For this review, take the finished solid that the model builds, in its own axes (mm). Face numbers are marked on the shaded views. A direction names the side the tool comes from. Coordinates: 2 decimals unless noted, no trailing zeros. Write each loop counter-clockwise with the first axis right and the second up, starting at its lowest first coordinate (ties: lowest second). Pieces come first, ordered by that corner, then holes. Notation, with made-up numbers: (69, 47.5) - (91, 47.5) arc R20 cw to (91, 70.5) - close; hole circle Ø3 at (81, 15). An arc over 180 degrees is marked (long way). Write each question's results on one line, items separated by ' | '.
Autodesk Inventor part; units mm, degrees
ref_plane "YZ Plane" through (0, 0, 0) normal (1, 0, 0) x (0, 1, 0)
ref_plane "XZ Plane" through (0, 0, 0) normal (0, 1, 0) x (-1, 0, 0)
ref_plane "XY Plane" through (0, 0, 0) normal (0, 0, 1) x (1, 0, 0)
sketch "Boceto1" plane through (0, 0, 0) normal (0, 0, 1) x (1, 0, 0)
  line L0 (64, 24) -> (64, 0)
  line L1 (0, 0) -> (0, 24)
  line L2 (0, 0) -> (0, 24) construction
  line L3 (40, 7) -> (40, 16)
  line L4 (64, 0) -> (64, 24)
  line L5 (0, 24) -> (0, 0)
  line L6 (64, 0) -> (64, 16)
  line L7 (40, 16) -> (24, 16)
  line L8 (0, 16) -> (0, 0)
  line L9 (24, 16) -> (40, 16)
  line L10 (64, 16) -> (64, 7)
  line L11 (0, 7) -> (0, 16)
  line L12 (48, 0) -> (48, 7)
  line L13 (16, 7) -> (16, 0)
  line L14 (24, 16) -> (24, 7)
  line L15 (48, 7) -> (40, 7)
  line L16 (24, 7) -> (16, 7)
  arc A0 (45.1449, 45.122) -> (18.8863, 45.1669) centre (32, 36) ccw
  circle A1 centre (32, 36) radius 8
  line L17 (64, 24) -> (59.8026, 24)
  line L18 (4.09, 24) -> (0, 24)
  line L19 (64, 0) -> (48, 0)
  line L20 (16, 0) -> (0, 0)
  line L21 (0, 0) -> (16, 0)
  line L22 (48, 0) -> (60.5696, 0)
  line L23 (0, 0) -> (16, 0)
  line L24 (48, 0) -> (64, 0)
  line L25 (0, 0) -> (16, 0)
  line L26 (48, 0) -> (64, 0)
  line L27 (4.09, 24) -> (18.8863, 45.1669)
  line L28 (45.1449, 45.122) -> (59.8026, 24)
  line L29 (16, 0) -> (48, 0)
  line L30 (0, 0) -> (64, 0)
  line L31 (64, 0) -> (64, 24)
  line L32 (32.0546, 51.9999) -> (31.9454, 51.9999)
  line L33 (0, 24) -> (0, 0)
  line L34 (0, 0) -> (64, 0)
  line L35 (64, 0) -> (64, 53.4326)
  line L36 (64, 53.4326) -> (0, 53.4326)
  line L37 (0, 53.4326) -> (0, 0)
  circle A2 centre (32, 36) radius 8
  point P0 (30.2848, 0)
  dimension "d6" = 24
  dimension "d9" = 32
  dimension "d10" = 16
  dimension "d11" = 9
sketch "Boceto2" plane through (0, 0, 0) normal (1, 0, 0) x (0, 1, 0)
  point P0 (0, 0)
sketch "Boceto3" plane through (0, 0, 0) normal (1, 0, 0) x (0, 1, 0)
  point P0 (0, 0)
sketch "Boceto4" plane through (0, 0, 0) normal (1, 0, 0) x (0, 1, 0)
  line L0 (0, 0) -> (0, -144)
  line L1 (0, -144) -> (36, -144)
  line L2 (0, -144) -> (16, -144)
  line L3 (16, -118) -> (16, -22)
  line L4 (16, 0) -> (0, 0)
  line L5 (0, 0) -> (0, -144)
  line L6 (36, -144) -> (16, -144)
  line L7 (16, -118) -> (52, -118)
  line L8 (52, -118) -> (52, -128)
  line L9 (36, -144) -> (52, -128)
  line L10 (52, 0) -> (16, 0)
  line L11 (16, -22) -> (52, -22)
  line L12 (52, -22) -> (52, 0)
  line L13 (52, -128) -> (52, -118)
  line L14 (52, -22) -> (52, 0)
  dimension "d15" = 144
  dimension "d17" = 16
  dimension "d22" = 22
extrude "Extrusión1" add sketch "Boceto4" along normal blind 64
extrude "Extrusión3" cut sketch "Boceto1" against normal blind 100 contours L17 L28 A0 L27 L18 L37 L36 L35
extrude "Extrusión4" cut sketch "Boceto1" against normal blind 100 contours A1
extrude "Extrusión5" cut sketch "Boceto1" against normal blind 144 contours L29 L13 L16 L14 L7 L3 L15 L12
fillet "Empalme1" radius 3 2 edges at (59.8026, 24, -11) (4.09, 24, -11)
properties part number "Pieza2 Base" material "Hierro, fundido"
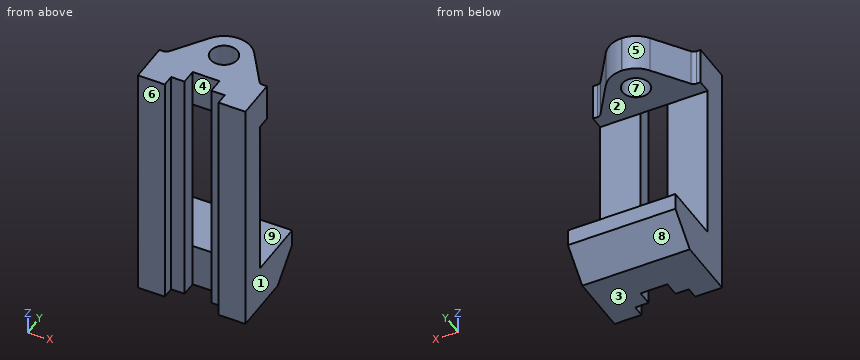
Q1. Take a section at C-C on y = 29.5. State the section outline as (x, z) points, plus the area to 3 significant figures.
Results found:
outline: (0, -144) - (64, -144) - (64, -118) - (0, -118) - close; (7.93, -22) - (27.34, -22) - (27.34, 0) - (7.93, 0) - close; (36.66, -22) - (55.99, -22) - (55.99, 0) - (36.66, 0) - close | area: 2,520 mm2
Q2. For the marked faces 1, 2, 3, 4 and 5, list the 3-axis set-ups (+Z, -Z, +X, -X, +Y, -Y) from which the entire face can be reached by the end or side of a thin tool; tool diameter is ignored.
Results found:
face 1: +Z, -Z, +X, +Y, -Y | face 2: +X, -X, +Y | face 3: -Z, +X, -X, +Y, -Y | face 4: +Z, -Z, -Y | face 5: +Z, -X, +Y
Q3. Wall thickness on line 1 along X through (y, z) = (10.5, -57); line 2 along Z through (x, y) = (21.5, 25); line 3 along Y through (x, z) = (32, -8.25): over which ranges is each line inside the solid? List them lowest first. Write a range as from..to.
Results found:
line 1: 0..24, 40..64 | line 2: -144..-118, -22..0 | line 3: 16..28, 44..52
Q4. For pin 1 (4 mm diameter, centred on x = 26, z = -19.5, fed in from +Y); pin 2 (14.5 mm diameter, centred on x = 32, y = 36, fed in from +Z); pin 3 (2 mm diameter, centred on x = 63.5, z = -9, fed in from +Y), all flat-tipped, find the tip position at first contact; note any pin that passes through.
Results found:
pin 1: y = 51.49 | pin 2: z = -118 | pin 3: y = 24
Q5. Take a section at B-B on z = -100. State the section outline as (x, y) points.
Results found:
outline: (0, 0) - (16, 0) - (16, 7) - (24, 7) - (24, 16) - (0, 16) - close; (40, 7) - (48, 7) - (48, 0) - (64, 0) - (64, 16) - (40, 16) - close
Q6. Take a section at A-A on x = 35.5. State the section outline as (y, z) points.
Results found:
outline: (16, -144) - (36, -144) - (52, -128) - (52, -118) - (16, -118) - close; (16, -22) - (28.81, -22) - (28.81, 0) - (16, 0) - close; (43.19, -22) - (51.61, -22) - (51.61, 0) - (43.19, 0) - close
Q7. Take a section at D-D on x = 10. State the section outline as (y, z) points, plus the area to 3 significant figures.
Results found:
outline: (0, -144) - (36, -144) - (52, -128) - (52, -118) - (16, -118) - (16, -22) - (32.45, -22) - (32.45, 0) - (0, 0) - close | area: 3,470 mm2
Q8. Mouldability with a two-part tool opening along Y and no side actions: class the marked faces 6, 7, 8 and 9 as pulls with the +Y half, pulls with the -Y half, needs draft (parallel to the pull), parting line crosses it, or undercut.
Results found:
face 6: pulls with the -Y half | face 7: undercut | face 8: pulls with the +Y half | face 9: needs draft
